```python
from build123d import *

# Parameters (mm, degrees)
SKETCH1_R           = 0.55
BOSS_EXTRUDE1_DEPTH = 1
BOSS_EXTRUDE3_DEPTH = 1.1
BOSS_EXTRUDE4_DEPTH = 1.25
SKETCH5_R           = 0.375
BOSS_EXTRUDE5_DEPTH = 0.05
SKETCH6_R           = 0.25
BOSS_EXTRUDE6_DEPTH = 0.05
CHAMFER1_SIZE       = 0.75
CHAMFER1_SIZE_2     = 0.5
MIRROR1_START       = -1.1
MIRROR1_DEPTH       = 1.1
MIRROR1_START_2     = -1.8
MIRROR1_2_DEPTH     = 2.5
MIRROR1_START_3     = 6.27611275
MIRROR1_3_OUTLINE_R = 0.375
MIRROR1_3_DEPTH     = 0.05
MIRROR1_START_4     = 6.32611275
MIRROR1_4_OUTLINE_R = 0.25
MIRROR1_4_DEPTH     = 0.05
FILLET2_R           = 0.05
BOSS_EXTRUDE7_DEPTH = 1
FILLET3_R           = 0.1


with BuildPart() as part:
    # Sketch1 → Boss-Extrude1 (new body)
    with BuildSketch(Plane(origin=(0, 0, 0), x_dir=(1, 0, 0), z_dir=(0, 1, 0))):
        with BuildLine():
            Line((-3, -1.6), (-1.799182122, 0.873466479))
            ThreePointArc((-1.799182122, 0.873466479), (0, 2), (1.799182122, 0.873466479))
            Line((1.799182122, 0.873466479), (3, -1.6))
            Line((3, -1.6), (-3, -1.6))
        make_face()
        with Locations(Location((0, 0, 0), (0, 0, 270))):
            Circle(SKETCH1_R, mode=Mode.SUBTRACT)
    extrude(amount=BOSS_EXTRUDE1_DEPTH)

    # Sketch3 → Boss-Extrude3 (add)
    with BuildSketch(Plane(origin=(0, 0, 0), x_dir=(-1, 0, 0), z_dir=(0, -1, 0))):
        with BuildLine():
            Line((2.514520254, -0.6), (3.412657784, -2.45))
            ThreePointArc((3.412657784, -2.45), (3.562510993, -2.875016795), (3.613323348, -3.322803983))
            Line((3.613323348, -3.322803983), (3.613323348, -6.273765877))
            Line((3.613323348, -6.273765877), (2.863323348, -7.572803983))
            Line((2.863323348, -7.572803983), (1.851870719, -6.988841535))
            Line((1.851870719, -6.988841535), (2.445398453, -5.960821345))
            Line((2.445398453, -5.960821345), (2.445398453, -3.322803983))
            ThreePointArc((2.445398453, -3.322803983), (2.424281128, -3.13670618), (2.362002989, -2.960071623))
            Line((2.362002989, -2.960071623), (1.701715763, -1.6))
            Line((1.701715763, -1.6), (2.514520254, -0.6))
        make_face()
    extrude(amount=BOSS_EXTRUDE3_DEPTH)

    # Sketch4 → Boss-Extrude4 (add, symmetric)
    with BuildSketch(Plane(origin=(2.003180044, -0.55, 0.513767997), x_dir=(1, 0, 0), z_dir=(0, 1, 0))):
        Polygon((-3.84639051, -6.470073538), (-4.875163646, -7.064035986), (-4.375163646, -7.930061389), (-3.34639051, -7.336098942), align=None)
    extrude(amount=BOSS_EXTRUDE4_DEPTH, both=True)

    # Sketch5 → Boss-Extrude5 (add)
    with BuildSketch(Plane(origin=(-5.435273078, 0, 3.138056375), x_dir=(0.5000000000000009, 0, 0.8660254037844383), z_dir=(-0.8660254037844382, 0, 0.5000000000000008))):
        with Locations((5.626578953, -0.55)):
            Circle(SKETCH5_R)
    extrude(amount=BOSS_EXTRUDE5_DEPTH)

    # Sketch6 → Boss-Extrude6 (add)
    with BuildSketch(Plane(origin=(-5.478574348, 0, 3.163056375), x_dir=(0.5000000000000008, 0, 0.8660254037844383), z_dir=(-0.8660254037844382, 0, 0.5000000000000007))):
        with Locations((5.626578953, -0.55)):
            Circle(SKETCH6_R)
    extrude(amount=BOSS_EXTRUDE6_DEPTH)

    # Chamfer1
    # the kernel refuses this chamfer: 0.75, 0.5 mm, written as the material it takes off along each edge
    with BuildSketch(Plane(origin=(-1.701715763, 0, 1.6), x_dir=(-0.43673323969900685, 0, 0.899591061172803), z_dir=(0, -1, 0))) as chamfer1_piece_1:
        Polygon((CHAMFER1_SIZE, 0), (-CHAMFER1_SIZE_2 * 0.422618261741, CHAMFER1_SIZE_2 * 0.906307787037), (0, 0), align=None)
    extrude(amount=3.043103543, mode=Mode.SUBTRACT)

    # Mirror1: read off the stored shape, not the designer's step
    # Mirror1 outline → Mirror1 (add)
    with BuildSketch(Plane(origin=(0, 0, 0), x_dir=(1, 0, 0), z_dir=(0, 1, 0)).offset(MIRROR1_START)):
        with BuildLine():
            Line((3.412657784, -2.45), (2.514520254, -0.6))
            Line((2.514520254, -0.6), (2.174766969, -1.01800124))
            Line((2.174766969, -1.01800124), (1.920082383, -2.049795531))
            Line((1.920082383, -2.049795531), (2.362002989, -2.960071623))
            ThreePointArc((2.362002989, -2.960071623), (2.424281128, -3.13670618), (2.445398453, -3.322803983))
            Line((2.445398453, -3.322803983), (2.445398453, -5.960821345))
            Line((2.445398453, -5.960821345), (1.851870719, -6.988841535))
            Line((1.851870719, -6.988841535), (1.843210465, -6.983841535))
            Line((1.843210465, -6.983841535), (1.343210465, -7.849866939))
            Line((1.343210465, -7.849866939), (2.371983602, -8.443829386))
            Line((2.371983602, -8.443829386), (2.871983602, -7.577803983))
            Line((2.871983602, -7.577803983), (2.863323348, -7.572803983))
            Line((2.863323348, -7.572803983), (3.613323348, -6.273765877))
            Line((3.613323348, -6.273765877), (3.613323348, -3.322803983))
            ThreePointArc((3.613323348, -3.322803983), (3.562510993, -2.875016795), (3.412657784, -2.45))
        make_face()
    extrude(amount=MIRROR1_DEPTH)

    # Mirror1 2 outline → Mirror1 2 (add)
    with BuildSketch(Plane(origin=(0, 0, 0), x_dir=(1, 0, 0), z_dir=(0, 1, 0)).offset(MIRROR1_START_2)):
        Polygon((2.871983602, -7.577803983), (1.843210465, -6.983841535), (1.343210465, -7.849866939), (2.371983602, -8.443829386), align=None)
    extrude(amount=MIRROR1_2_DEPTH)

    # Mirror1 3 outline → Mirror1 3 (add)
    with BuildSketch(Plane(origin=(0, 0, 0), x_dir=(0.500000000000001, 0, -0.866025403784438), z_dir=(0.866025403784438, 0, 0.500000000000001)).offset(MIRROR1_START_3)):
        with Locations((-5.626578953, -0.55)):
            Circle(MIRROR1_3_OUTLINE_R)
    extrude(amount=MIRROR1_3_DEPTH)

    # Mirror1 4 outline → Mirror1 4 (add)
    with BuildSketch(Plane(origin=(0, 0, 0), x_dir=(0.500000000000001, 0, -0.866025403784438), z_dir=(0.866025403784438, 0, 0.500000000000001)).offset(MIRROR1_START_4)):
        with Locations((-5.626578953, -0.55)):
            Circle(MIRROR1_4_OUTLINE_R)
    extrude(amount=MIRROR1_4_DEPTH)

    # Fillet2
    fillet2_edges = [part.edges().sort_by_distance(p)[0] for p in [
        (-2.852784872, -0.55, 7.711057158),
        (-2.833586142, -0.55, 7.844310334),
    ]]
    fillet(fillet2_edges, radius=FILLET2_R - 0.0001)  # a hair under: the kernel refuses the full size

    # Sketch7 → Boss-Extrude7 (add)
    with BuildSketch(Plane(origin=(0, 0, 0), x_dir=(1, 0, 0), z_dir=(0, 1, 0))):
        Polygon((-0.8, -2.6), (0.8, -2.6), (1.3, -1.6), (0, -0.8), (-1.3, -1.6), align=None)
    extrude(amount=BOSS_EXTRUDE7_DEPTH)

    # Fillet3
    # the kernel refuses this fillet: 0.1 mm, written as the material it takes off along each edge
    with BuildSketch(Plane(origin=(2.871983602, -1.1, 7.577803983), x_dir=(-0.8660254028383251, 0, -0.5000000016387168), z_dir=(0, 1, 0))) as fillet3_piece_1_section:
        with BuildLine():
            CenterArc((FILLET3_R * 0.9999999985, FILLET3_R), FILLET3_R, 180.000000086, 89.999999914)
            Line((-FILLET3_R * 1.50001067123e-09, FILLET3_R * 0.9999999985), (0, 0))
            Line((0, 0), (FILLET3_R * 0.9999999985, 0))
        make_face()
    fillet3_piece_1 = extrude(amount=1.1, mode=Mode.PRIVATE)
    fillet3_piece_1 = split(fillet3_piece_1, bisect_by=Plane(origin=(2.863323348, -1.1, 7.572803983), z_dir=(0.8660254038383292, 0, 0.49999999990665916)), keep=Keep.TOP, mode=Mode.PRIVATE)
    add(fillet3_piece_1, mode=Mode.SUBTRACT)
    with BuildSketch(Plane(origin=(2.371983602, 0.95, 8.443829386), x_dir=(0.5000000003396727, 0, -0.8660254035883286), z_dir=(0, -1, 0)), Plane(origin=(1.343210465, -2.05, 7.849866939), x_dir=(0.4999999999066601, 0, -0.8660254038383285), z_dir=(0, 1, 0)), Plane(origin=(-2.371983602, -2.05, 8.443829386), x_dir=(-0.5000000000000007, 0, -0.8660254037844383), z_dir=(0, 1, 0))) as fillet3_piece_2:
        with BuildLine():
            CenterArc((FILLET3_R, -FILLET3_R), FILLET3_R, 90, 89.999999953)
            Line((0, -FILLET3_R), (0, 0))
            Line((0, 0), (FILLET3_R, 0))
        make_face()
    extrude(amount=3, mode=Mode.SUBTRACT)
    with BuildSketch(Plane(origin=(-2.871983602, -2.05, 7.577803983), x_dir=(0.5000000000000002, 0, 0.8660254037844386), z_dir=(0, 1, 0))) as fillet3_piece_3_section:
        with BuildLine():
            CenterArc((FILLET3_R, FILLET3_R), FILLET3_R, 180, 90)
            Line((0, FILLET3_R), (0, 0))
            Line((0, 0), (FILLET3_R, 0))
        make_face()
    fillet3_piece_3 = extrude(amount=3, mode=Mode.PRIVATE)
    fillet3_piece_3 = split(fillet3_piece_3, bisect_by=Plane(origin=(-2.871983602, -1.1, 7.577803983), z_dir=(0, -1, 0)), keep=Keep.TOP, mode=Mode.PRIVATE)
    fillet3_piece_3 = split(fillet3_piece_3, bisect_by=Plane(origin=(-2.863323348, -2.05, 7.572803983), z_dir=(-0.8660254037844362, 0, 0.5000000000000044)), keep=Keep.TOP, mode=Mode.PRIVATE)
    add(fillet3_piece_3, mode=Mode.SUBTRACT)
    with BuildSketch(Plane(origin=(-2.871983602, -2.05, 7.577803983), x_dir=(0.5000000000000002, 0, 0.8660254037844386), z_dir=(0, 1, 0))) as fillet3_piece_4_section:
        with BuildLine():
            CenterArc((FILLET3_R, FILLET3_R), FILLET3_R, 180, 90)
            Line((0, FILLET3_R), (0, 0))
            Line((0, 0), (FILLET3_R, 0))
        make_face()
    fillet3_piece_4 = extrude(amount=3, mode=Mode.PRIVATE)
    fillet3_piece_4 = split(fillet3_piece_4, bisect_by=Plane(origin=(-2.871983602, -1.1, 7.577803983), z_dir=(0, -1, 0)), keep=Keep.TOP, mode=Mode.PRIVATE)
    fillet3_piece_4 = split(fillet3_piece_4, bisect_by=Plane(origin=(-2.863323348, -2.05, 7.572803983), z_dir=(0.8660254037844362, 0, -0.5000000000000044)), keep=Keep.TOP, mode=Mode.PRIVATE)
    add(fillet3_piece_4, mode=Mode.SUBTRACT)
    with BuildSketch(Plane(origin=(-2.871983602, -2.05, 7.577803983), x_dir=(0.5000000000000002, 0, 0.8660254037844386), z_dir=(0, 1, 0))) as fillet3_piece_5_section:
        with BuildLine():
            CenterArc((FILLET3_R, FILLET3_R), FILLET3_R, 180, 90)
            Line((0, FILLET3_R), (0, 0))
            Line((0, 0), (FILLET3_R, 0))
        make_face()
    fillet3_piece_5 = extrude(amount=3, mode=Mode.PRIVATE)
    fillet3_piece_5 = split(fillet3_piece_5, bisect_by=Plane(origin=(-2.871983602, 0, 7.577803983), z_dir=(0, -1, 0)), keep=Keep.TOP, mode=Mode.PRIVATE)
    fillet3_piece_5 = split(fillet3_piece_5, bisect_by=Plane(origin=(-2.871983602, -1.1, 7.577803983), z_dir=(0, 1, 0)), keep=Keep.TOP, mode=Mode.PRIVATE)
    fillet3_piece_5 = split(fillet3_piece_5, bisect_by=Plane(origin=(-2.863323348, -2.05, 7.572803983), z_dir=(-0.8660254037844362, 0, 0.5000000000000044)), keep=Keep.TOP, mode=Mode.PRIVATE)
    add(fillet3_piece_5, mode=Mode.SUBTRACT)
    with BuildSketch(Plane(origin=(-2.871983602, -2.05, 7.577803983), x_dir=(0.5000000000000002, 0, 0.8660254037844386), z_dir=(0, 1, 0))) as fillet3_piece_6_section:
        with BuildLine():
            CenterArc((FILLET3_R, FILLET3_R), FILLET3_R, 180, 90)
            Line((0, FILLET3_R), (0, 0))
            Line((0, 0), (FILLET3_R, 0))
        make_face()
    fillet3_piece_6 = extrude(amount=3, mode=Mode.PRIVATE)
    fillet3_piece_6 = split(fillet3_piece_6, bisect_by=Plane(origin=(-2.871983602, 0, 7.577803983), z_dir=(0, 1, 0)), keep=Keep.TOP, mode=Mode.PRIVATE)
    fillet3_piece_6 = split(fillet3_piece_6, bisect_by=Plane(origin=(-2.863323348, -2.05, 7.572803983), z_dir=(-0.8660254037844362, 0, 0.5000000000000044)), keep=Keep.TOP, mode=Mode.PRIVATE)
    add(fillet3_piece_6, mode=Mode.SUBTRACT)
    with BuildSketch(Plane(origin=(-2.871983602, -2.05, 7.577803983), x_dir=(0.5000000000000002, 0, 0.8660254037844386), z_dir=(0, 1, 0))) as fillet3_piece_7_section:
        with BuildLine():
            CenterArc((FILLET3_R, FILLET3_R), FILLET3_R, 180, 90)
            Line((0, FILLET3_R), (0, 0))
            Line((0, 0), (FILLET3_R, 0))
        make_face()
    fillet3_piece_7 = extrude(amount=3, mode=Mode.PRIVATE)
    fillet3_piece_7 = split(fillet3_piece_7, bisect_by=Plane(origin=(-2.871983602, 0, 7.577803983), z_dir=(0, 1, 0)), keep=Keep.TOP, mode=Mode.PRIVATE)
    fillet3_piece_7 = split(fillet3_piece_7, bisect_by=Plane(origin=(-2.863323348, -2.05, 7.572803983), z_dir=(0.8660254037844362, 0, -0.5000000000000044)), keep=Keep.TOP, mode=Mode.PRIVATE)
    add(fillet3_piece_7, mode=Mode.SUBTRACT)
    with BuildSketch(Plane(origin=(-1.343210465, 0.95, 7.849866939), x_dir=(-0.8660254037844438, 0, 0.4999999999999912), z_dir=(0, -1, 0))) as fillet3_piece_8:
        with BuildLine():
            CenterArc((FILLET3_R, FILLET3_R), FILLET3_R, 180, 90)
            Line((0, FILLET3_R), (0, 0))
            Line((0, 0), (FILLET3_R, 0))
        make_face()
    extrude(amount=3, mode=Mode.SUBTRACT)
    with BuildSketch(Plane(origin=(2.871983602, -2.05, 7.577803983), x_dir=(-0.866025403632075, 0, -0.5000000002639015), z_dir=(0, 1, 0)), Plane(origin=(2.871983602, 0, 7.577803983), x_dir=(-0.866025403632075, 0, -0.5000000002639015), z_dir=(0, 1, 0))) as fillet3_piece_9:
        with BuildLine():
            CenterArc((FILLET3_R, FILLET3_R), FILLET3_R, 179.999999995, 90.000000005)
            Line((0, FILLET3_R), (0, 0))
            Line((0, 0), (FILLET3_R, 0))
        make_face()
    extrude(amount=0.95, mode=Mode.SUBTRACT)


solid = part.part
```
Verification items for the finished model (mm, model axes). A direction names the side the tool comes from. Coordinates: 2 decimals unless noted, no trailing zeros. Order: outer loops, then holes, each group sorted by start corner. A loop starts at its lowest first (then second) coordinate and runs counter-clockwise, first axis right, second up. Notation, with made-up numbers: (14, 17.5) -> (63, 17.5) arc R19 ccw to (63, 33.5) -> close; hole circle Ø10 at (32, -17.75). An arc over 180 degrees is marked (long way). Answer as CSV lines item,"result". Start each with the question number.
1) Cross-section at A-A, the plane y = 0.3. Record the boundary of the cut face in (x, z), then the cut area to 3 significant figures.
2) Material ranges on L1, parallel to X at y = -0.2, z = 3.75; L2, parallel to Y at x = 2.25, z = 2.25; L3, parallel to Y at x = 2.5, z = 1.5, recorded low to high. Write a range as [from, to].
3) Cross-section at D-D, the plane x = -1. Record the boundary of the cut face in (y, z).
4) Cross-section at C-C, the plane z = 5.75. Record the boundary of the cut face in (x, y).
5) Gauge pin test, flat ends, axial feed: pin 1 Ø1.3 at (x, z) = (0, 0) entering from -Y; pin 2 Ø1.9 at (x, z) = (-2.5, 5) entering from +Y; pin 3 Ø0.5 at (x, z) = (3, 4.5) entering from -Y; pin 4 Ø0.5 at (x, y) = (-2.5, 0.5) entering from +Z. Record the tip position at first contact, or that the pin passes through.
6) Cross-section at B-B, the plane x = 0. Record the boundary of the cut face in (y, z), then the cut area to 3 significant figures.
7) Set-up check for faces 4 (the face through (-2.445, -0.5, 4.7)), 5 (the face through (1.852, -0.568, 8.143)), 6 (the face through (0, 0, 1)): record each of +Z, -Z, +X, -X, +Y, -Y from which the full face is reachable in a straight line by a thin tool's end or side.
8) Release check for a two-part mould opening along Z. For faces 1 (the face through (1.046, 0.493, 2.107)), 2 (the face through (0.545, 0.493, -0.072)), 3 (the face through (-2, 0.7, 8)) record: released by +Z, released by -Z, zero draft, split by the parting line, or undercut.
Conclusion:
1,outline,"(-3, 1.6) -> (-1.8, -0.87) arc R2 ccw to (1.8, -0.87) -> (3, 1.6) -> (1.3, 1.6) -> (0.8, 2.6) -> (-0.8, 2.6) -> (-1.3, 1.6) -> close; (-2.82, 7.66) arc R0.1 ccw to (-2.79, 7.53) -> (-1.84, 6.98) -> (-1.39, 7.76) arc R0.1 ccw to (-1.43, 7.9) -> (-2.29, 8.39) arc R0.1 ccw to (-2.42, 8.36) -> close; (1.39, 7.76) -> (1.84, 6.98) -> (2.79, 7.53) arc R0.1 ccw to (2.82, 7.66) -> (2.42, 8.36) arc R0.1 ccw to (2.29, 8.39) -> (1.43, 7.9) arc R0.1 ccw to start; hole circle Ø1.1 at (0, 0)"
1,area,"18.3 mm²"
2,L1,"x = [-3.61, -2.45], [2.45, 3.61]"
2,L2,"y = [-1.1, 0]"
2,L3,"y = [-1.1, 1]"
3,outline,"(0, -1.73) -> (1, -1.73) -> (1, 2.2) -> (0, 2.2) -> close"
4,outline,"(-3.61, -1.1) -> (-2.45, -1.1) -> (-2.45, 0) -> (-3.61, 0) -> close; (2.45, -1.1) -> (3.61, -1.1) -> (3.61, 0) -> (2.45, 0) -> close"
5,pin 1,"stops at y = 0"
5,pin 2,"stops at y = 0"
5,pin 3,"stops at y = -1.1"
5,pin 4,"stops at z = 8.41"
6,outline,"(0, -2) -> (1, -2) -> (1, -0.55) -> (0, -0.55) -> close; (0, 0.55) -> (1, 0.55) -> (1, 2.6) -> (0, 2.6) -> close"
6,area,"3.50 mm²"
7,face 4,"+Y, -Y"
7,face 5,"+Z, +Y, -Y"
7,face 6,"-Z, -Y"
8,face 1,"released by +Z"
8,face 2,"undercut"
8,face 3,"zero draft"
